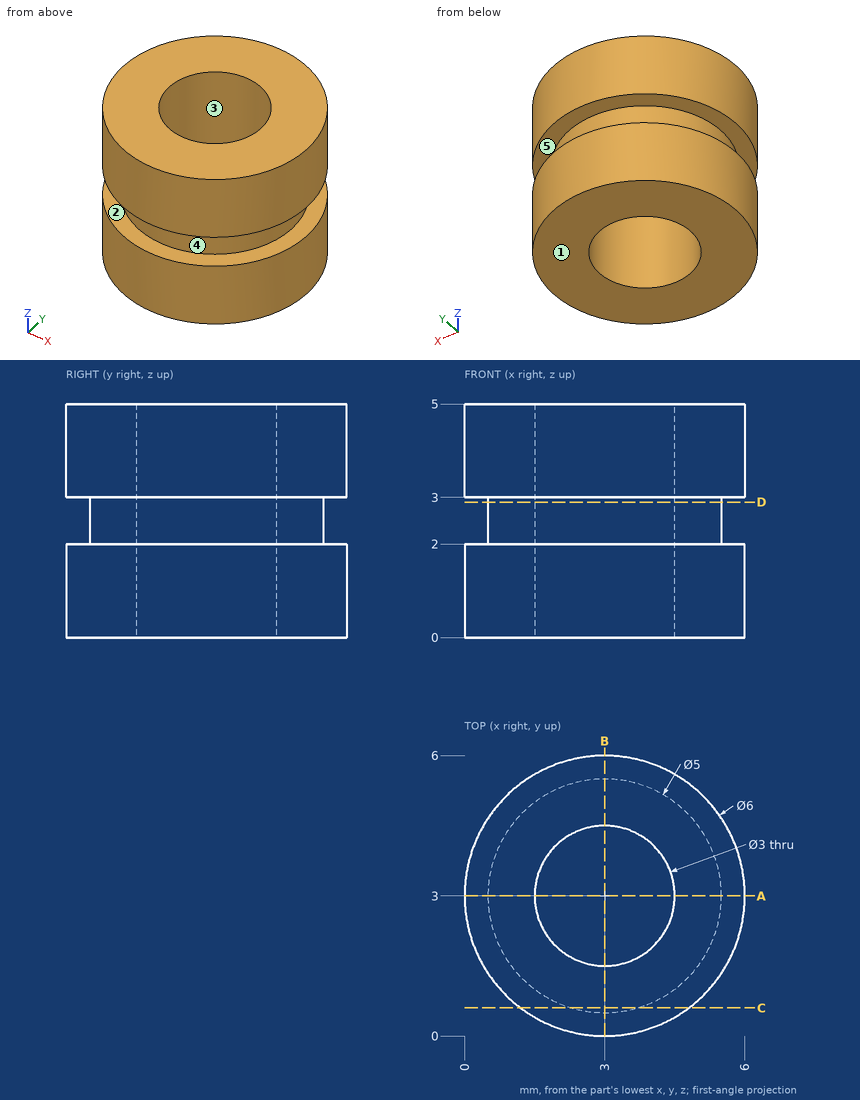
Here's the drawing with two shaded views (mm, measured from the low corner). I have some questions. A direction names the side the tool comes from. Give positions to 0.01 mm unless a question says otherwise; leave off trailing zeros. Loops run counter-clockwise (first coordinate to the right, second up) from the corner with the lowest first, then second, coordinate; pieces in that order, holes last. Notation, with made-up numbers: (86.5, -0.75) -> (103.5, -0.75) arc R9 cw to (103.5, 5.25) -> close; hole circle Ø3 at (51.5, 1.25). An arc over 180 degrees is marked (long way). One line per item, written item: value.
Q1. Suppose I cut it at C-C on y = 0.6. Please give me the cut outline in (x, z).
Answers follow:
outline: (1.2, 0) -> (4.8, 0) -> (4.8, 2) -> (3.7, 2) -> (3.7, 3) -> (4.8, 3) -> (4.8, 5) -> (1.2, 5) -> (1.2, 3) -> (2.3, 3) -> (2.3, 2) -> (1.2, 2) -> close
Q2. Suppose I cut it at D-D on z = 2.9. Please give me the cut outline in (x, y), then the cut area to 3 significant figures.
Answers follow:
outline: circle Ø5 at (3, 3); hole circle Ø3 at (3, 3)
area: 12.6 mm^2
Q3. Suppose I cut it at A-A on y = 3. Please give me the cut outline in (x, z), then the cut area to 3 significant figures.
Answers follow:
outline: (0, 0) -> (1.5, 0) -> (1.5, 5) -> (0, 5) -> (0, 3) -> (0.5, 3) -> (0.5, 2) -> (0, 2) -> close; (4.5, 0) -> (6, 0) -> (6, 2) -> (5.5, 2) -> (5.5, 3) -> (6, 3) -> (6, 5) -> (4.5, 5) -> close
area: 14.0 mm^2
Q4. If I drill on line 1 along Y through (x, z) = (3, 2.85); line 2 along Y through (x, z) = (3, 3.3); line 3 along Z through (x, y) = (1.25, 0.7), over which ranges is the centre line in solid material (lowest first)?
Answers follow:
line 1: 0.5 to 1.5, 4.5 to 5.5
line 2: 0 to 1.5, 4.5 to 6
line 3: 0 to 2, 3 to 5
Q5. We'd pull the mould along Y, two halves only. Please class the marked faces 3, 4 and 5: pulls with the +Y half, pulls with the -Y half, needs draft (parallel to the pull), parting line crosses it, or undercut.
Answers follow:
face 3: undercut
face 4: parting line crosses it
face 5: needs draft
Q6. I'm going to push flat-ended pins straight in: pin 1 Ø1 at (x, z) = (1.5, 4) entering from -Y; pin 2 Ø1.5 at (y, z) = (4, 4) entering from +X; pin 3 Ø1.5 at (y, z) = (1, 1) entering from +X. Where does each tip first touch, or does it pass through?
Answers follow:
pin 1: y = 0.17
pin 2: x = 5.99
pin 3: x = 5.73
Q7. On a 3-axis mill with a long thin cutter (end or side, diameter ignored), from which of +Z, -Z, +X, -X, +Y, -Y can I reach the whole of each face in a straight line? I mean the marked faces 1 and 2. Say none if no direction works.
Answers follow:
face 1: -Z, +X, -X, +Y, -Y
face 2: none
